The model under review builds one solid part; all positions refer to its coordinate system, in mm. A direction names the side the tool comes from. Round coordinates to 2 decimals unless told otherwise and drop trailing zeros. Order: outer loops, then holes, each group sorted by start corner. A loop starts at its lowest first (then second) coordinate and runs counter-clockwise, first axis right, second up.
```python
from build123d import *

# Parameters (mm, degrees)
CYLINDER004_R     = 1.55
CYLINDER004_DEPTH = 10
CYLINDER003_R     = 3.5
CYLINDER003_DEPTH = 3.5


with BuildPart() as bolt_hole_cylinder:
    # Cylinder004 → Cylinder004 (new body)
    with BuildSketch(Plane.XY):
        Circle(CYLINDER004_R)
    extrude(amount=CYLINDER004_DEPTH)


with BuildPart() as hole_extraction:
    # Cylinder003 → Cylinder003 (new body)
    with BuildSketch(Plane.XY):
        Circle(CYLINDER003_R)
    extrude(amount=CYLINDER003_DEPTH)

    # Fusion003: union bolt hole cylinder
    add(bolt_hole_cylinder.part)


with BuildPart() as bolt_cover:
    # Cone → Cone (revolve)
    with BuildSketch(Plane.XZ):
        Polygon((0, 0), (5, 0), (4, 12), (0, 12), align=None)
    revolve(axis=Axis((0, 0, 0), (0, 0, 1)))

    # Cut001: cut hole extraction
    add(hole_extraction.part, mode=Mode.SUBTRACT)


solid = bolt_cover.part
```
(1) To check wall thickness, follow probe 1 along Z at (x, y) = (-2, 2.5); probe 2 along Y at (x, z) = (0, 1.3); probe 3 along X at (y, z) = (-0.75, 8.75). State the ranges of each line that lie inside material, in increasing order.
Data:
probe 1: z = 3.5 to 12
probe 2: y = -4.89 to -3.5, 3.5 to 4.89
probe 3: x = -4.2 to -1.36, 1.36 to 4.2
(2) Consider section D-D (z = 1). Write out the cut boundary in (x, y).
Data:
outline: circle Ø9.83 at (0, 0); hole circle Ø7 at (0, 0)
(3) Consider section A-A (x = 0). Write out the cut boundary in (y, z), and give its area (4 significant figures).
Data:
outline: (-5, 0) - (-3.5, 0) - (-3.5, 3.5) - (-1.55, 3.5) - (-1.55, 10) - (1.55, 10) - (1.55, 3.5) - (3.5, 3.5) - (3.5, 0) - (5, 0) - (4, 12) - (-4, 12) - close
area: 63.35 mm2
(4) Insertion check: pin 1 (2 mm diameter, centred on x = 0, y = 0, fed in from -Z); pin 2 (6 mm diameter, centred on x = -1, z = 3, fed in from -Y); pin 3 (3 mm diameter, centred on x = 0.5, z = 7, fed in from +Y). Each pin has a flat end and moves straight along its axis. Give the tip position at first contact, or say it passes through.
Data:
pin 1: stops at z = 10
pin 2: stops at y = -4.99
pin 3: stops at y = 4.54
(5) Draft analysis for pull direction X (two halves, no side actions). For faces 1 (the flat face through (0, 0, 10)), 2 (the conical face through (-4.49, 0.2, 6.08)), 3 (the flat face through (-2.2, -3.3, 0)), state which applies: pulls with the +X half, pulls with the -X half, needs draft (parallel to the pull), parting line crosses it, or undercut.
Data:
face 1: undercut
face 2: parting line crosses it
face 3: needs draft
(6) Consider section C-C (z = 6). Write out the cut boundary in (x, y), and give its area (3 significant figures).
Data:
outline: circle Ø9 at (0, 0); hole circle Ø3.1 at (0, 0)
area: 56.1 mm2
(7) For faces 4 (the flat face through (0, 0, 12)), 5 (the cylindrical face through (0.715, -1.375, 6.704)), list the 3-axis set-ups (+Z, -Z, +X, -X, +Y, -Y) from which the entire face can be reached by the end or side of a thin tool; tool diameter is ignored.
Data:
face 4: +Z, +X, -X, +Y, -Y
face 5: -Z
